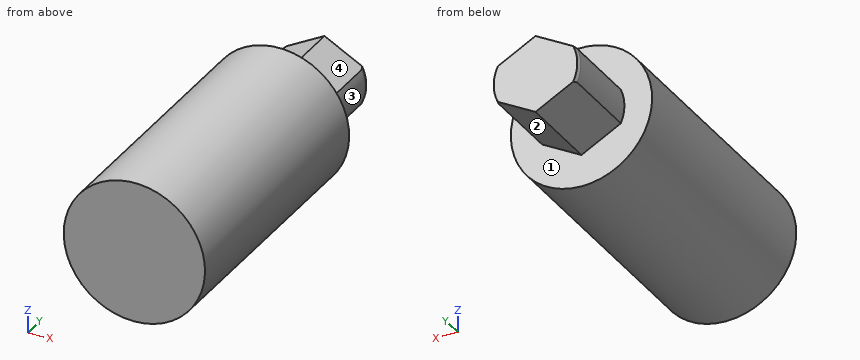
```python
from build123d import *

# Parameters (mm, degrees)
SKETCH_1_R          = 10.0871205
EXTRUDE_1_DEPTH     = 20.174241
SKETCH_2_R          = 16.5871205
EXTRUDE_2_DEPTH     = 63.26
CHAMFER_1_SIZE      = 1
CHAMFER_1_SIZE2     = 0.267949192
SKETCH_4_OUTSIDE_W  = 54.318
SKETCH_4_OUTSIDE_H  = 54.318
CUT_EXTRUDE_2_DEPTH = 20.174241


with BuildPart() as part:
    # Sketch 1 → Extrude 1 (new body)
    with BuildSketch(Plane(origin=(0, 0, 0), x_dir=(1, 0, 0), z_dir=(0, 1, 0))):
        with Locations(Location((0, 0, 0), (0, 0, 270))):
            Circle(SKETCH_1_R)
    extrude(amount=EXTRUDE_1_DEPTH)

    # Sketch 2 → Extrude 2 (add)
    with BuildSketch(Plane.XZ):
        with Locations(Location((0, 0, 0), (0, 0, 270))):
            Circle(SKETCH_2_R)
    extrude(amount=EXTRUDE_2_DEPTH)

    # Chamfer 1
    chamfer_1_edges = [part.edges().sort_by_distance(p)[0] for p in [
        (0, 20.174241, -10.0871205),
    ]]
    chamfer_1_side = [part.faces().sort_by_distance(p)[0] for p in [
        (0, 10.0871205, -10.0871205),
    ]]
    chamfer(chamfer_1_edges, length=CHAMFER_1_SIZE, length2=CHAMFER_1_SIZE2, reference=chamfer_1_side[0])

    # Sketch 4 outside → Cut-Extrude 2 (cut)
    with BuildSketch(Plane(origin=(0, 20.174241, 0), x_dir=(1, 0, 0), z_dir=(0, 1, 0))):
        Rectangle(SKETCH_4_OUTSIDE_W, SKETCH_4_OUTSIDE_H)
        with BuildLine():
            Line((-9.244998647, 4.0348482), (0, 9.07840845))
            Line((0, 9.07840845), (9.244998647, 4.0348482))
            ThreePointArc((9.244998647, 4.0348482), (10.0871205, 0), (9.244998647, -4.0348482))
            Line((9.244998647, -4.0348482), (0, -9.07840845))
            Line((0, -9.07840845), (-9.244998647, -4.0348482))
            ThreePointArc((-9.244998647, -4.0348482), (-10.0871205, 0), (-9.244998647, 4.0348482))
        make_face(mode=Mode.SUBTRACT)
    extrude(amount=-CUT_EXTRUDE_2_DEPTH, mode=Mode.SUBTRACT)


solid = part.part
```
Could you check a few things on this model? Use its own coordinates, in mm. Face numbers are marked on the shaded views. A direction names the side the tool comes from. Give positions to 0.01 mm unless a question says otherwise; leave off trailing zeros. Order: outer loops, then holes, each group sorted by start corner. A loop starts at its lowest first (then second) coordinate and runs counter-clockwise, first axis right, second up.
Q1. Suppose I cut it at B-B, the plane x = -7. Write out the boundary of the cut face in (y, z).
Q2. Suppose I cut it at D-D, the plane x = -2. Write out the boundary of the cut face in (y, z), and give its area (3 significant figures).
Q3. If I drill on line 1 along Y through (x, z) = (-15, 0); line 2 along X through (y, z) = (-38, -0.5); line 3 along Z through (x, y) = (-2, -54.5), over which ranges is the centre line in solid material (lowest first)?
Q4. Suppose I cut it at C-C, the plane y = -22. Write out the boundary of the cut face in (x, z).
Q5. I'm going to push flat-ended pins straight in: P1, Ø4, axis at x = 6.5, z = 8.5, coming from the +Y side; P2, Ø8, axis at x = -12.5, y = -54.5, coming from the -Z side; P3, Ø3, axis at y = -45.5, z = 5.5, coming from the -X side. Where does each tip first touch, or does it pass through?
Q6. Suppose I cut it at A-A, the plane z = 0. Write out the boundary of the cut face in (x, y).
Q7. For the marked faces 1, 2, 3 and 4, which set-ups out of +Z, -Z, +X, -X, +Y, -Y let a thin tool reach every point of the face, with its end or its side?
Solution:
1. outline: (-63.26, -15.04) - (0, -15.04) - (0, -5.26) - (20.17, -5.26) - (20.17, 5.26) - (0, 5.26) - (0, 15.04) - (-63.26, 15.04) - close
2. outline: (-63.26, -16.47) - (0, -16.47) - (0, -7.99) - (20.17, -7.99) - (20.17, 7.99) - (0, 7.99) - (0, 16.47) - (-63.26, 16.47) - close
2. area: 2,410 mm2
3. line 1: y = -63.26 to 0
3. line 2: x = -16.58 to 16.58
3. line 3: z = -16.47 to 16.47
4. outline: circle Ø33.17 at (0, 0)
5. P1: stops at y = 0
5. P2: stops at z = -14.24
5. P3: stops at x = -16.1
6. outline: (-16.59, -63.26) - (16.59, -63.26) - (16.59, 0) - (10.09, 0) - (10.09, 19.17) - (9.82, 20.17) - (-9.82, 20.17) - (-10.09, 19.17) - (-10.09, 0) - (-16.59, 0) - close
7. face 1: +Y
7. face 2: -Z, +X, +Y
7. face 3: +X, +Y
7. face 4: +Z, +X, +Y
